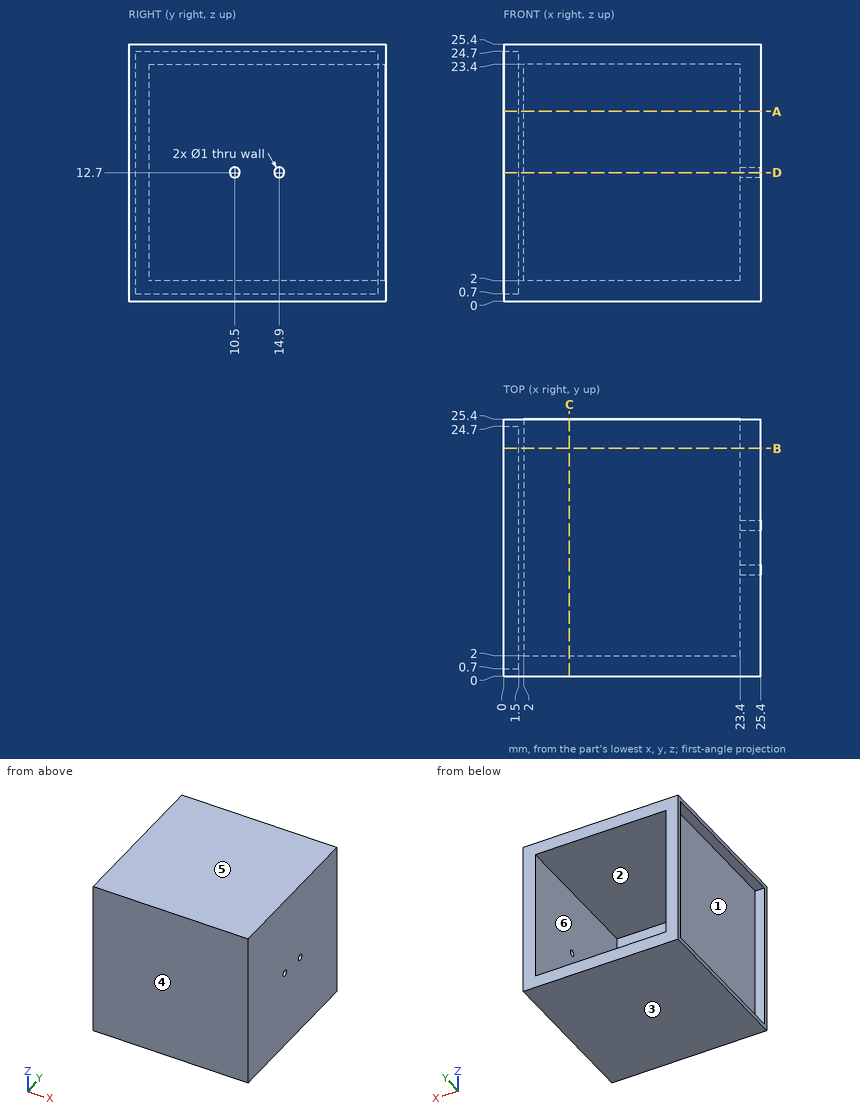
Here's the drawing with two shaded views (mm, measured from the low corner). I have some questions. A direction names the side the tool comes from. Give positions to 0.01 mm unless a question says otherwise; leave off trailing zeros. Write each loop counter-clockwise with the first axis right and the second up, starting at its lowest first coordinate (ties: lowest second). Pieces come first, ordered by that corner, then holes. Notation, with made-up numbers: (44.5, 53.5) -> (73.5, 53.5) arc R31 ccw to (73.5, 92.5) -> close; hole circle Ø10 at (11, 75). An arc over 180 degrees is marked (long way). Use one line per item in the form item = value. Start each with the question number.
1. On a 3-axis mill with a long thin cutter (end or side, diameter ignored), from which of +Z, -Z, +X, -X, +Y, -Y can I reach the whole of each face in a straight line? I mean the marked faces 1, 2 and 3. Say none if no direction works.
2. Imagine slicing it at D-D on z = 12.7. List the corners of the cut face in (x, y) for me, plus the area to 3 significant figures.
3. Imagine slicing it at A-A on z = 18.75. List the corners of the cut face in (x, y) for me, plus the area to 3 significant figures.
4. Imagine slicing it at B-B on y = 22.5. List the corners of the cut face in (x, z) for me.
5. If I drill on L1, parallel to Y at x = 24.45, z = 12.7; L2, parallel to X at y = 4, z = 10; L3, parallel to Z at x = 20, y = 5, over which ranges is the centre line in solid material (lowest first)?
6. Will these pins go through, and if not, where does the flat tip stop? pin 1 Ø1.5 at (x, z) = (9.5, 20) entering from +Y; pin 2 Ø7 at (y, z) = (13.5, 9) entering from -X.
7. Imagine slicing it at C-C on x = 6.5. List the corners of the cut face in (y, z) for me.
8. Thinking about a two-plate mould opening in Z: for the marked faces 4, 5 and 6, which applies, +Z half, -Z half, draft (parallel to the pull), parting line (faces both ways), or undercut?
Entries:
q1.face_1 = -X
q1.face_2 = +Y
q1.face_3 = -Z, +X, -X, +Y, -Y
q2.outline = (0, 0) -> (25.4, 0) -> (25.4, 10) -> (23.4, 10) -> (23.4, 2) -> (2, 2) -> (2, 25.4) -> (0, 25.4) -> (0, 24.7) -> (1.5, 24.7) -> (1.5, 0.7) -> (0, 0.7) -> close; (23.4, 11) -> (25.4, 11) -> (25.4, 14.4) -> (23.4, 14.4) -> close; (23.4, 15.4) -> (25.4, 15.4) -> (25.4, 25.4) -> (23.4, 25.4) -> close
q2.area = 104 mm²
q3.outline = (0, 0) -> (25.4, 0) -> (25.4, 25.4) -> (23.4, 25.4) -> (23.4, 2) -> (2, 2) -> (2, 25.4) -> (0, 25.4) -> (0, 24.7) -> (1.5, 24.7) -> (1.5, 0.7) -> (0, 0.7) -> close
q3.area = 108 mm²
q4.outline = (0, 0) -> (25.4, 0) -> (25.4, 25.4) -> (0, 25.4) -> (0, 24.7) -> (1.5, 24.7) -> (1.5, 0.7) -> (0, 0.7) -> close; hole (2, 2) -> (23.4, 2) -> (23.4, 23.4) -> (2, 23.4) -> close
q5.L1 = 0 to 10, 11 to 14.4, 15.4 to 25.4
q5.L2 = 1.5 to 2, 23.4 to 25.4
q5.L3 = 0 to 2, 23.4 to 25.4
q6.pin_1 = 2
q6.pin_2 = 1.5
q7.outline = (0, 0) -> (25.4, 0) -> (25.4, 2) -> (2, 2) -> (2, 23.4) -> (25.4, 23.4) -> (25.4, 25.4) -> (0, 25.4) -> close
q8.face_4 = draft
q8.face_5 = +Z half
q8.face_6 = undercut
